Verification items for the finished model (mm, model axes). Give positions to 0.01 mm unless a question says otherwise; leave off trailing zeros. Loops run counter-clockwise (first coordinate to the right, second up) from the corner with the lowest first, then second, coordinate; pieces in that order, holes last. Notation, with made-up numbers: M 60.25,85.5 L 92.25,85.5 A25 cw 92.25,114.5 Z; hole C 46,-28 d6. An arc over 180 degrees is marked long. Use a Markdown table: item, result.
Autodesk Inventor part; units mm, degrees
ref_plane "YZ Plane" through (0, 0, 0) normal (1, 0, 0) x (0, 1, 0)
ref_plane "XZ Plane" through (0, 0, 0) normal (0, 1, 0) x (-1, 0, 0)
ref_plane "XY Plane" through (0, 0, 0) normal (0, 0, 1) x (1, 0, 0)
sketch "Sketch1" plane through (0, 0, 0) normal (1, 0, 0) x (0, 1, 0)
  circle A0 centre (0, 0) radius 34.75
  circle A1 centre (-6.9, 0) radius 5
  dimension "d0" = 69.5
  dimension "d1" = 10
  dimension "d2" = 6.9
extrude "Extrusion1" add sketch "Sketch1" along normal blind 2
sketch "Sketch2" plane through (2, 0, 0) normal (1, 0, 0) x (0, 0, -1)
  circle A0 centre (0, 0) radius 30
  point P0 (0, 30)
  dimension "d5" = 60
hole "Hole1" at (2, 30, 0) direction (-1, 0, 0) diameter 4.3 depth 10
pattern_circular "Circular Pattern1" count 12 over 360 about axis through (0, 0, 0) along (1, 0, 0) of "Hole1"
sketch "Sketch3" plane through (2, 0, 0) normal (1, 0, 0) x (0, 0, -1)
  circle A0 centre (0, -6.9) radius 5
  circle A1 centre (0, -6.9) radius 7
  point P0 (0, 0)
  point P1 (0, 0.1)
  dimension "d16" = 14
hole "Hole2" at (2, 0.1, 0) direction (-1, 0, 0) diameter 2.2 depth 10
pattern_circular "Circular Pattern2" count 4 over 360 about axis through (0, -6.9, 0) along (1, 0, 0) of "Hole2"
properties part number "sample-transfer_plate" material "ABS Plastic orange"
(1) Cross-section at D-D on z = 15. Record the cut outline in (x, y).
Results below:
| item | result |
|---|---|
| outline | M 0,-31.35 L 2,-31.35 L 2,-28.13 L 0,-28.13 Z; M 0,-23.83 L 2,-23.83 L 2,23.83 L 0,23.83 Z; M 0,28.13 L 2,28.13 L 2,31.35 L 0,31.35 Z |
(2) Cross-section at B-B on y = 30. Record the cut outline in (x, z), then the cut area to 4 significant figures.
Results below:
| item | result |
|---|---|
| outline | M 0,-17.54 L 2,-17.54 L 2,-2.15 L 0,-2.15 Z; M 0,2.15 L 2,2.15 L 2,17.54 L 0,17.54 Z |
| area | 61.55 mm^2 |
(3) Gauge pin test, flat ends, axial feed: P1, Ø3, axis at y = -6.9, z = -7, coming from the -X side; P2, Ø1, axis at x = 0.5, y = 21.5, coming from the +Z side. Record the tip position at first contact, or that the pin passes through.
Results below:
| item | result |
|---|---|
| P1 | x = 0 |
| P2 | z = 27.69 |
(4) Cross-section at C-C on y = -6.9. Record the cut outline in (x, z).
Results below:
| item | result |
|---|---|
| outline | M 0,-34.06 L 2,-34.06 L 2,-8.1 L 0,-8.1 Z; M 0,-5.9 L 2,-5.9 L 2,-5 L 0,-5 Z; M 0,5 L 2,5 L 2,5.9 L 0,5.9 Z; M 0,8.1 L 2,8.1 L 2,34.06 L 0,34.06 Z |
(5) Draft check along Y on faces 1 (the flat face through (0, 7, 0)), 2 (the cylindrical face through (0.99, 18.68, -29.3)), 3 (the cylindrical face through (1, -13.9, -1.1)), 4 (the cylindrical face through (0.99, -1.16, -28.19)). Enter one of: +Y half, -Y half, draft (parallel to the pull), parting line (faces both ways), or undercut.
Results below:
| item | result |
|---|---|
| face 1 | draft |
| face 2 | parting line |
| face 3 | undercut |
| face 4 | undercut |
(6) Material ranges on line 1 (Y direction, x = 0.35, z = 26); line 2 (Y direction, x = 0.75, z = -24.5); line 3 (Z direction, x = 0.35, y = -5), recorded low to high.
Results below:
| item | result |
|---|---|
| line 1 | -23.06 to -17.15, -12.85 to 12.85, 17.15 to 23.06 |
| line 2 | -24.64 to -16.56, -13.44 to 13.44, 16.56 to 24.64 |
| line 3 | -34.39 to -4.62, 4.62 to 34.39 |
(7) Cross-section at A-A on z = -7. Record the cut outline in (x, y), then the cut area to 3 significant figures.
Results below:
| item | result |
|---|---|
| outline | M 0,-34.04 L 2,-34.04 L 2,-8 L 0,-8 Z; M 0,-5.8 L 2,-5.8 L 2,34.04 L 0,34.04 Z |
| area | 132 mm^2 |
